Verification items for this drawing (mm, ordinates from the low corner). A direction names the side the tool comes from. Coordinates: 2 decimals unless noted, no trailing zeros. Order: outer loops, then holes, each group sorted by start corner. A loop starts at its lowest first (then second) coordinate and runs counter-clockwise, first axis right, second up. Notation, with made-up numbers: M -30,65.5 L -16,65.5 A11 ccw -16,73.5 Z; hole C 22.5,-27.5 d9. An arc over 180 degrees is marked long. Return JSON: item names as keys, results as strings. Group by question number.
1. Section check A-A, the plane y = 2.5. Record the cut outline in (x, z).
2. Section check C-C, the plane z = 3. Record the cut outline in (x, y).
3. Set-up check for the marked faces 1, 2 and 3: record each of +Z, -Z, +X, -X, +Y, -Y from which the full face is reachable in a straight line by a thin tool's end or side.
4. Gauge pin test, flat ends, axial feed: pin 1 (2 mm diameter, centred on y = 1.5, z = 10.5, fed in from +X); pin 2 (2 mm diameter, centred on x = 4.5, z = 19, fed in from +Y). Record the tip position at first contact, or that the pin passes through.
5. Section check D-D, the plane z = 26. Record the cut outline in (x, y), plus the area to 3 significant figures.
6. Material ranges on line 1 along Z through (x, y) = (3.1, 4.5); line 2 along X through (y, z) = (2.3, 15.5); line 3 along Y through (x, z) = (2.55, 44.5), recorded low to high.
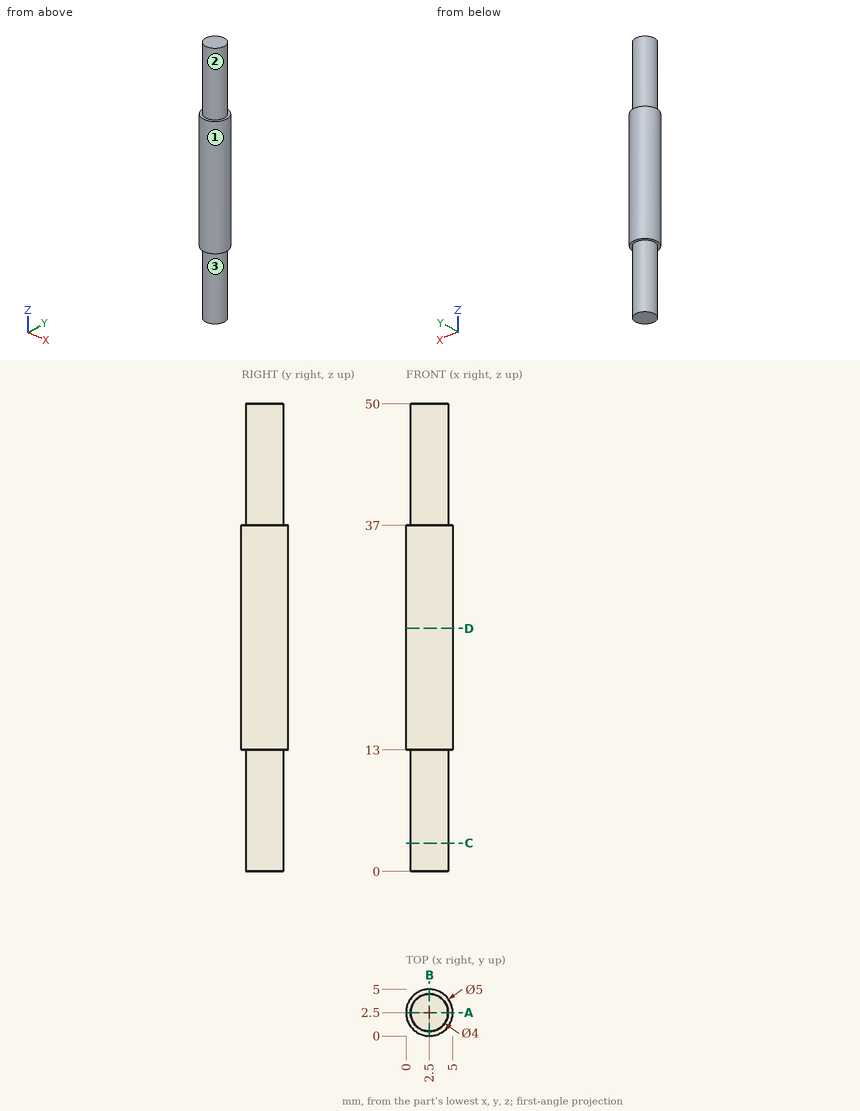
Answers follow:
{
 "1": {"outline": "M 0,13 L 0.5,13 L 0.5,0 L 4.5,0 L 4.5,13 L 5,13 L 5,37 L 4.5,37 L 4.5,50 L 0.5,50 L 0.5,37 L 0,37 Z"},
 "2": {"outline": "C 2.5,2.5 d4"},
 "3": {"face 1": "+Z, -Z", "face 2": "+Z", "face 3": "-Z"},
 "4": {"pin 1": "x = 4.5", "pin 2": "y = 4.79"},
 "5": {"outline": "C 2.5,2.5 d5", "area": "19.6 mm^2"},
 "6": {"line 1": "13 to 37", "line 2": "0.01 to 4.99", "line 3": "0.5 to 4.5"}
}
